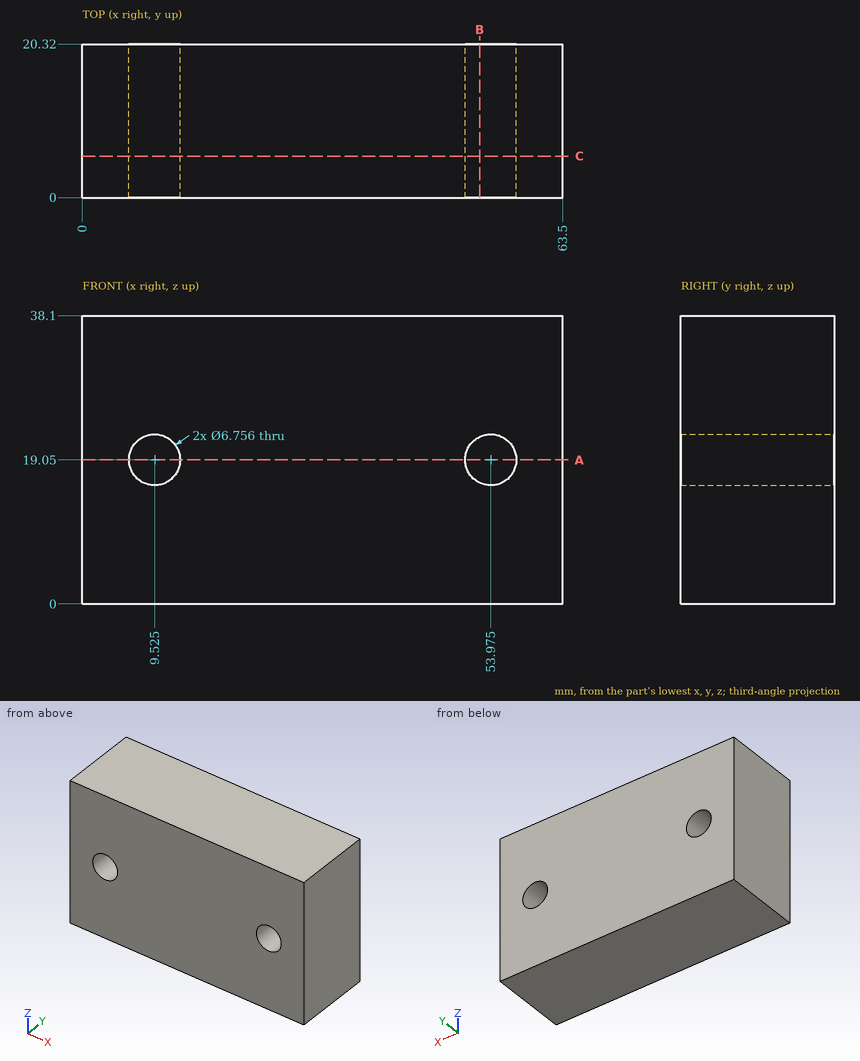
Geometry: see drawing. Coordinates: mm, zero at the bounding-box minimum. Round coordinates to 2 decimals unless told otherwise and drop trailing zeros. Loops run counter-clockwise (first coordinate to the right, second up) from the corner with the lowest first, then second, coordinate; pieces in that order, holes last. Notation, with made-up numbers: M -10,-33 L 22,-33 A24 cw 22,-16 Z; hole C 28,-20.5 d9. An arc over 180 degrees is marked long. Use a Markdown table: item, result. Add a question column.
1. Cut plane B-B, the plane x = 52.5. Output: boundary loops of the cut face in (y, z), and give its area (3 significant figures).
2. Contact query for a flat-ended pin moving along its axis: pin 1 (6 mm diameter, centred on x = 9.525, z = 19.05, fed in from -Y). Output: stop coordinate, or through.
3. Cut plane A-A, the plane z = 19.05. Output: boundary loops of the cut face in (x, y).
4. Ray query, line 1 along X through (y, z) = (18, 19.5); line 2 along Z through (x, y) = (52.5, 1.5); line 3 along Z through (x, y) = (10, 19) (1 decimal). Return the intervals inside material, ascending. Write a range as [from, to].
5. Cut plane C-C, the plane y = 5.5. State how many separate pieces and enclosed holes the cut face has, and give its area (3 significant figures).
Solution:
| question | item | result |
|---|---|---|
| 1 | outline | M 0,0 L 20.32,0 L 20.32,16.01 L 0,16.01 Z; M 0,22.09 L 20.32,22.09 L 20.32,38.1 L 0,38.1 Z |
| 1 | area | 651 mm2 |
| 2 | pin 1 | passes through |
| 3 | outline | M 0,0 L 6.15,0 L 6.15,20.32 L 0,20.32 Z; M 12.9,0 L 50.6,0 L 50.6,20.32 L 12.9,20.32 Z; M 57.35,0 L 63.5,0 L 63.5,20.32 L 57.35,20.32 Z |
| 4 | line 1 | x = [0, 6.18], [12.87, 50.63], [57.32, 63.5] |
| 4 | line 2 | z = [0, 16.01], [22.09, 38.1] |
| 4 | line 3 | z = [0, 15.7], [22.4, 38.1] |
| 5 | separate pieces | 1 |
| 5 | enclosed holes | 2 |
| 5 | area | 2,350 mm2 |
